For this review, take the finished solid that the model builds, in its own axes (mm). Face numbers are marked on the shaded views. A direction names the side the tool comes from. Give positions to 0.01 mm unless a question says otherwise; leave off trailing zeros. Write each loop counter-clockwise with the first axis right and the second up, starting at its lowest first coordinate (ties: lowest second). Pieces come first, ordered by that corner, then holes. Notation, with made-up numbers: (15, 31) -> (47, 31) arc R11 cw to (47, 35) -> close; hole circle Ø2 at (83, -31). An arc over 180 degrees is marked (long way). Return JSON: item names as keys, results as strings.
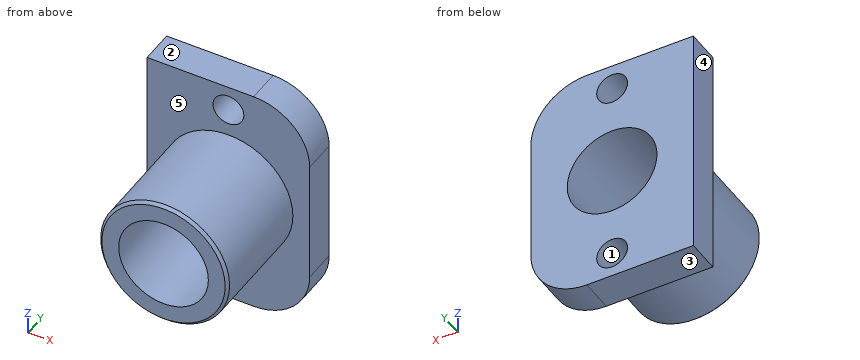
from build123d import *

# Parameters (mm, degrees)
F0_R     = 2.75
F1_DEPTH = 6
F2_R     = 11.5
F3_DEPTH = 20
F4_R     = 8
F5_DEPTH = 26.001
F6_SIZE  = 0.5


with BuildPart() as f1:
    # F0 (on Front) → F1 (new body)
    with BuildSketch(Plane.XZ):
        with BuildLine():
            Line((0, 42), (0, 0))
            Line((0, 0), (19, 0))
            ThreePointArc((19, 0), (26.071068, 2.928932), (29, 10))
            Line((29, 10), (29, 32))
            ThreePointArc((29, 32), (26.071068, 39.071068), (19, 42))
            Line((19, 42), (0, 42))
        make_face()
        with Locations((14.5, 4.5)):
            Circle(F0_R, mode=Mode.SUBTRACT)
        with Locations((14.5, 37.5)):
            Circle(F0_R, mode=Mode.SUBTRACT)
    extrude(amount=F1_DEPTH)

    # F2 (on face) → F3 (join)
    with BuildSketch(Plane.XZ.offset(6)):
        with Locations((14.5, 21)):
            Circle(F2_R)
    extrude(amount=F3_DEPTH)

    # F4 (on face) → F5 (cut, through all)
    with BuildSketch(Plane.XZ.offset(26)):
        with Locations((14.5, 21)):
            Circle(F4_R)
    extrude(amount=-F5_DEPTH, mode=Mode.SUBTRACT)

    # F6
    f6_edges = [f1.edges().sort_by_distance(p)[0] for p in [
        (3, -26, 21),
    ]]
    chamfer(f6_edges, length=F6_SIZE)


solid = f1.part
1. For the marked faces 4 and 5, list the 3-axis set-ups (+Z, -Z, +X, -X, +Y, -Y) from which the entire face can be reached by the end or side of a thin tool; tool diameter is ignored.
Results found:
{"face 4": "+Z, -Z, -X, +Y, -Y", "face 5": "-Y"}
2. Add section B-B, the plane x = 14.5. State the section outline as (y, z) points, plus the area to 3 significant figures.
Results found:
{"outline": "(-26, 10) -> (-25.5, 9.5) -> (-6, 9.5) -> (-6, 7.25) -> (0, 7.25) -> (0, 13) -> (-26, 13) -> close; (-26, 29) -> (0, 29) -> (0, 34.75) -> (-6, 34.75) -> (-6, 32.5) -> (-25.5, 32.5) -> (-26, 32) -> close; (-6, 0) -> (0, 0) -> (0, 1.75) -> (-6, 1.75) -> close; (-6, 40.25) -> (0, 40.25) -> (0, 42) -> (-6, 42) -> close", "area": "230 mm²"}
3. The part is to be moulded in two halves that separate along Z. For the marked faces 1, 2 and 3, say which applies: +Z half, -Z half, draft (parallel to the pull), parting line (faces both ways), or undercut.
Results found:
{"face 1": "undercut", "face 2": "+Z half", "face 3": "-Z half"}
4. To check wall thickness, follow probe 1 along Z at (x, y) = (14.5, -1.7); probe 2 along Z at (x, y) = (14.5, -6.75); probe 3 along Y at (x, z) = (5, 32). State the ranges of each line that lie inside material, in increasing order.
Results found:
{"probe 1": "z = 0 to 1.75, 7.25 to 13, 29 to 34.75, 40.25 to 42", "probe 2": "z = 9.5 to 13, 29 to 32.5", "probe 3": "y = -6 to 0"}
5. Add section D-D, the plane z = 37.5. State the section outline as (x, y) points.
Results found:
{"outline": "(0, -6) -> (11.75, -6) -> (11.75, 0) -> (0, 0) -> close; (17.25, -6) -> (27.35, -6) -> (27.35, 0) -> (17.25, 0) -> close"}
6. Add section C-C, the plane y = -20.5. State the section outline as (x, z) points.
Results found:
{"outline": "circle Ø23 at (14.5, 21); hole circle Ø16 at (14.5, 21)"}
7. For pin 1 (1 mm diameter, centred on x = 14, z = 37.5, fed in from +Y); pin 2 (2 mm diameter, centred on y = -7.5, z = 25, fed in from -X); pin 3 (12 mm diameter, centred on x = 11.5, y = -21.5, fed in from -Z); pin 4 (12 mm diameter, centred on y = -21.5, z = 24.5, fed in from +X), all flat-tipped, find the tip position at first contact; note any pin that passes through.
Results found:
{"pin 1": "passes through", "pin 2": "stops at x = 3.4", "pin 3": "stops at z = 9.5", "pin 4": "stops at x = 26"}
8. Add section A-A, the plane z = 21. State the section outline as (x, y) points.
Results found:
{"outline": "(0, -6) -> (3, -6) -> (3, -25.5) -> (3.5, -26) -> (6.5, -26) -> (6.5, 0) -> (0, 0) -> close; (22.5, -26) -> (25.5, -26) -> (26, -25.5) -> (26, -6) -> (29, -6) -> (29, 0) -> (22.5, 0) -> close"}
